The drawing under review shows one solid part. Ordinate dimensions are in mm from its lowest x, y, z. A direction names the side the tool comes from. Coordinates: 2 decimals unless noted, no trailing zeros. Order: outer loops, then holes, each group sorted by start corner. A loop starts at its lowest first (then second) coordinate and runs counter-clockwise, first axis right, second up.
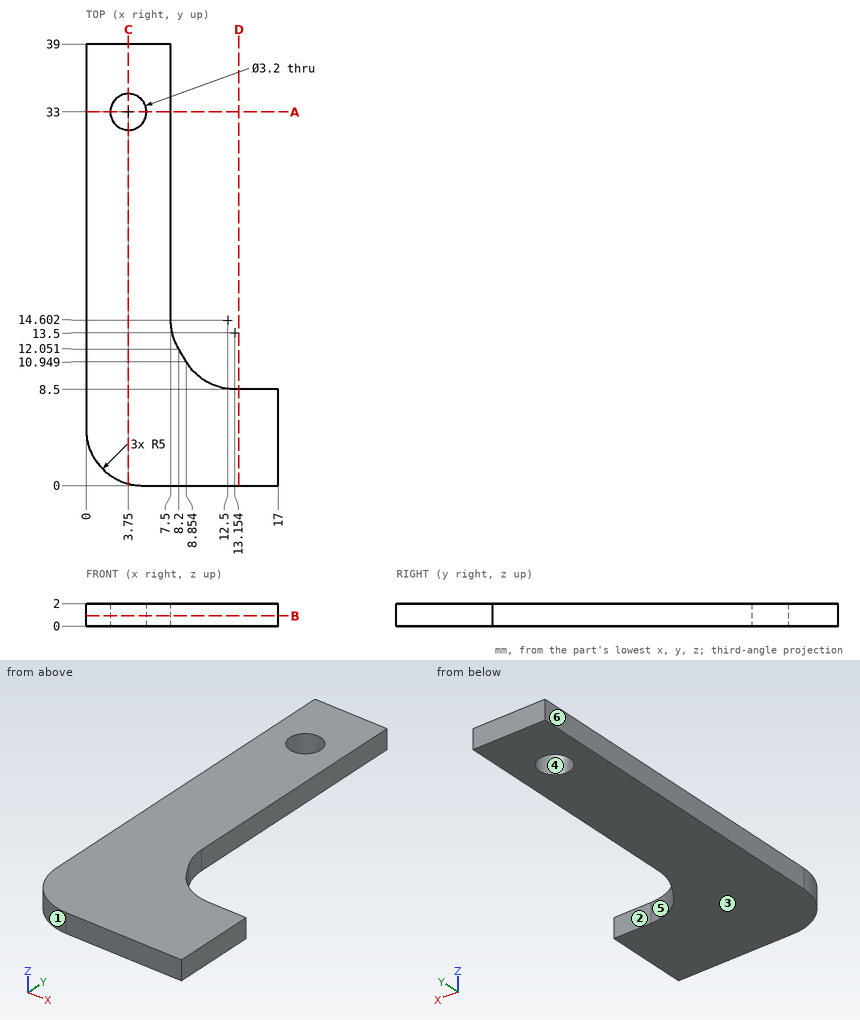
1. Machinability: for the marked faces 1 and 2, which of the approach directions +Z, -Z, +X, -X, +Y, -Y give a long, thin tool a straight path to every point of the face, cutting with its end or side? Answer none if there is none.
Answer below:
face 1: +Z, -Z, -X, -Y
face 2: +Z, -Z, +X, +Y
2. Take a section at A-A, the plane y = 33. Give the boundary of the cut face in (x, z).
Answer below:
outline: (0, 0) - (2.15, 0) - (2.15, 2) - (0, 2) - close; (5.35, 0) - (7.5, 0) - (7.5, 2) - (5.35, 2) - close
3. Take a section at D-D, the plane x = 13.5. Give the boundary of the cut face in (y, z), plus the area to 3 significant figures.
Answer below:
outline: (0, 0) - (8.5, 0) - (8.5, 2) - (0, 2) - close
area: 17.0 mm2
4. To check wall thickness, follow L1, parallel to X at y = 24, z = 1.15; L2, parallel to Y at x = 3.75, z = 1.35; L3, parallel to Y at x = 15.5, z = 0.85. State the ranges of each line that lie inside material, in increasing order.
Answer below:
L1: x = 0 to 7.5
L2: y = 0.16 to 31.4, 34.6 to 39
L3: y = 0 to 8.5
5. Take a section at C-C, the plane x = 3.75. Give the boundary of the cut face in (y, z).
Answer below:
outline: (0.16, 0) - (31.4, 0) - (31.4, 2) - (0.16, 2) - close; (34.6, 0) - (39, 0) - (39, 2) - (34.6, 2) - close
6. Clearance check with flat-ended pins moving along their axes: pin 1 Ø5 at (x, y) = (3.75, 33) entering from -Z; pin 2 Ø0.6 at (x, z) = (15.5, 1.5) entering from +Y; pin 3 Ø0.6 at (y, z) = (29.5, 1) entering from +X. State where each tip first meets the part, or that it passes through.
Answer below:
pin 1: stops at z = 0
pin 2: stops at y = 8.5
pin 3: stops at x = 7.5
7. The part is to be moulded in two halves that separate along X. For the marked faces 3, 4, 5 and 6, say which applies: +X half, -X half, draft (parallel to the pull), parting line (faces both ways), or undercut.
Answer below:
face 3: draft
face 4: undercut
face 5: +X half
face 6: -X half
8. Take a section at B-B, the plane z = 0.9. Give the boundary of the cut face in (x, y).
Answer below:
outline: (0, 5) arc R5 ccw to (5, 0) - (17, 0) - (17, 8.5) - (13.15, 8.5) arc R5 cw to (8.85, 10.95) - (8.2, 12.05) arc R5 cw to (7.5, 14.6) - (7.5, 39) - (0, 39) - close; hole circle Ø3.2 at (3.75, 33)
